```python
from build123d import *

# Parameters (mm, degrees)
BOSS_EXTRUDE1_DEPTH              = 57.15
F_1_2_0_5_DIAMETER_HOLE1_D       = 12.7
F_1_2_0_5_DIAMETER_HOLE1_DEPTH   = 45.72
F_1_2_0_5_DIAMETER_HOLE1_TIP     = 3.815464931
F_10_32_TAPPED_HOLE1_REACH       = 63.237
F_10_32_TAPPED_HOLE1_BORE_R      = 2.0193
F_29_0_136_DIAMETER_HOLE1_REACH  = 63.237
F_29_0_136_DIAMETER_HOLE1_BORE_R = 1.7272


with BuildPart() as part:
    # Sketch1 → Boss-Extrude1 (new body)
    with BuildSketch(Plane(origin=(0, 0, 0), x_dir=(1, 0, 0), z_dir=(0, 1, 0))):
        Polygon((5.499261314, -9.525), (10.998522628, 0), (5.499261314, 9.525), (-5.499261314, 9.525), (-10.998522628, 0), (-5.499261314, -9.525), align=None)
    extrude(amount=BOSS_EXTRUDE1_DEPTH)

    # 1/2 (0.5) Diameter Hole1
    with Locations(Plane(origin=(0, 0, 0), x_dir=(-1, 0, 0), z_dir=(0, -1, 0))):
        with Locations((0, 0)):
            Hole(F_1_2_0_5_DIAMETER_HOLE1_D / 2, depth=F_1_2_0_5_DIAMETER_HOLE1_DEPTH)
            with Locations((0, 0, -(F_1_2_0_5_DIAMETER_HOLE1_DEPTH + F_1_2_0_5_DIAMETER_HOLE1_TIP / 2))):  # 118° drill point
                Cone(0, F_1_2_0_5_DIAMETER_HOLE1_D / 2, F_1_2_0_5_DIAMETER_HOLE1_TIP, mode=Mode.SUBTRACT)

    # #10-32 Tapped Hole1 bore → #10-32 Tapped Hole1 (cut, up to next)
    with BuildSketch(Plane.XY.offset(9.525), mode=Mode.PRIVATE) as f_10_32_tapped_hole1_sk1:
        with Locations((0, 22.225)):
            Circle(F_10_32_TAPPED_HOLE1_BORE_R)
    f_10_32_tapped_hole1_tool1 = extrude(f_10_32_tapped_hole1_sk1.sketch, amount=-F_10_32_TAPPED_HOLE1_REACH, mode=Mode.PRIVATE) & part.part
    add(f_10_32_tapped_hole1_tool1.solids().sort_by_distance((0, 22.225, 9.525))[0], mode=Mode.SUBTRACT)

    # #29 (0.136) Diameter Hole1 bore → #29 (0.136) Diameter Hole1 (cut, up to next)
    with BuildSketch(Plane.XY.offset(9.525), mode=Mode.PRIVATE) as f_29_0_136_diameter_hole1_sk1:
        with Locations((0, 38.4175)):
            Circle(F_29_0_136_DIAMETER_HOLE1_BORE_R)
    f_29_0_136_diameter_hole1_tool1 = extrude(f_29_0_136_diameter_hole1_sk1.sketch, amount=-F_29_0_136_DIAMETER_HOLE1_REACH, mode=Mode.PRIVATE) & part.part
    add(f_29_0_136_diameter_hole1_tool1.solids().sort_by_distance((0, 38.4175, 9.525))[0], mode=Mode.SUBTRACT)


solid = part.part
```
Geometry check sheet. Reference: the model listing, model coordinates, mm. A direction names the side the tool comes from. Give positions to 0.01 mm unless a question says otherwise; leave off trailing zeros. Write each loop counter-clockwise with the first axis right and the second up, starting at its lowest first coordinate (ties: lowest second). Pieces come first, ordered by that corner, then holes.
1) Section check B-B, the plane z = 8. State how many separate pieces and enclosed holes the cut face has, and give its area (3 significant figures).
2) Material ranges on L1, parallel to Y at x = 0, z = 7.45; L2, parallel to Z at x = 0, y = 36.5 (3 decimals); L3, parallel to Z at x = 4.5, y = 36 (3 decimals), recorded low to high.
3) Section check A-A, the plane y = 33. Record the boundary of the cut face in (x, z) (3 decimals), and give its area (3 significant figures).
4) Access from +Z, -Z, +X, -X, +Y, -Y to the whole of each face (thin tool, end or side, straight path). Record for faces 4 (the cylindrical face through (1.595, 37.756, 7.838)), 5 (the flat face through (-0.2, 0, -6.5)).
5) Section check C-C, the plane x = -9.25. Record the boundary of the cut face in (y, z).
6) Release check for a two-part mould opening along Z. For faces 1 (the cylindrical face through (-2.017, 22.314, 7.793)), 2 (the flat face through (0, 28, 9.525)), 3 (the cylindrical face through (-0.8, 23.2, -6.3)) record: pulls with the +Z half, pulls with the -Z half, needs draft (parallel to the pull), parting line crosses it, or undercut.
7) Gauge pin test, flat ends, axial feed: pin 1 (1.5 mm diameter, centred on x = -3, z = -2.5, fed in from -Y); pin 2 (3 mm diameter, centred on y = 25.5, z = 3, fed in from +X); pin 3 (2 mm diameter, centred on x = 0, y = 38.42, fed in from +Z). Record the tip position at first contact, or that the pin passes through.
Computed:
1. separate pieces: 1
1. enclosed holes: 2
1. area: 707 mm2
2. L1: y = 0 to 20.21, 24.24 to 36.69, 40.14 to 57.15
2. L2: z = -9.525 to -6.35, 6.35 to 9.525
2. L3: z = -9.525 to -4.48, 4.48 to 9.525
3. outline: (-10.999, 0) - (-5.499, -9.525) - (5.499, -9.525) - (10.999, 0) - (5.499, 9.525) - (-5.499, 9.525) - close; hole circle Ø12.7 at (0, 0)
3. area: 188 mm2
4. face 4: +Z
4. face 5: +Z, -Z, +X, -X, -Y
5. outline: (0, -3.03) - (57.15, -3.03) - (57.15, 3.03) - (0, 3.03) - close
6. face 1: needs draft
6. face 2: pulls with the +Z half
6. face 3: undercut
7. pin 1: stops at y = 46.74
7. pin 2: stops at x = 10.13
7. pin 3: stops at z = -6.27
